Here's how the part is built. I have some questions about the finished solid (model axes, mm). Give positions to 0.01 mm unless a question says otherwise; leave off trailing zeros. Write each loop counter-clockwise with the first axis right and the second up, starting at its lowest first coordinate (ties: lowest second). Pieces come first, ordered by that corner, then holes. Notation, with made-up numbers: (-3, 67.5) -> (29, 67.5) arc R23 ccw to (29, 83.5) -> close; hole circle Ø9 at (56, -30.5). An arc over 180 degrees is marked (long way). Use one line per item in the form item = value.
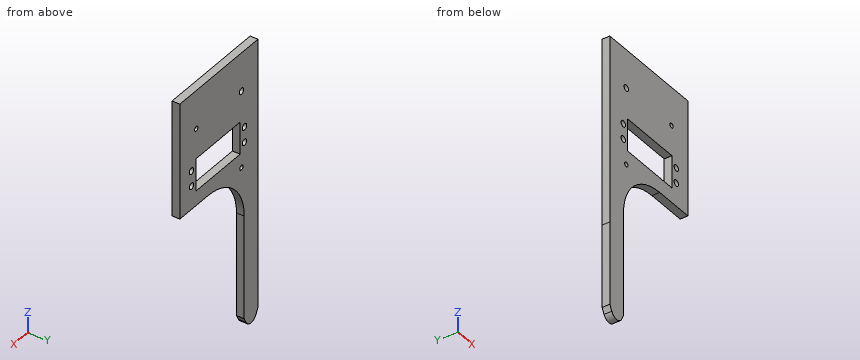
```python
from build123d import *

# Parameters (mm, degrees)
BOSS_EXTRUDE1_DEPTH = 2.5
SKETCH2_W           = 39
SKETCH2_H           = 19
CUT_EXTRUDE2_DEPTH  = 118.286651401
SKETCH6_R           = 1.5
SKETCH6_R_2         = 2
CUT_EXTRUDE11_DEPTH = 118.286651401
SKETCH8_W           = 39.164697568
SKETCH8_H           = 2
CUT_EXTRUDE12_DEPTH = 10
SKETCH9_W           = 40.5
SKETCH9_H           = 21
CUT_EXTRUDE14_DEPTH = 10
SKETCH10_R          = 2
CUT_EXTRUDE16_DEPTH = 10
SKETCH14_W          = 61.515702129
SKETCH14_H          = 51.963385976
CUT_EXTRUDE19_DEPTH = 10
FILLET4_R           = 5


with BuildPart() as part:
    # Sketch1 → Boss-Extrude1 (new, symmetric)
    with BuildSketch(Plane(origin=(0, 0, 0), x_dir=(1, 0, 0), z_dir=(0, 1, 0))):
        with BuildLine():
            Line((-45.466733516, 13.267794591), (-45.466733516, -107.999697871))
            Line((-45.466733516, -107.999697871), (25.786244138, -107.999697871))
            Line((25.786244138, -107.999697871), (25.786244138, -33))
            Line((25.786244138, -33), (0, -33))
            ThreePointArc((0, -33), (-23.334523779, -23.334523779), (-33, 0))
            Line((-33, 0), (-33, 13.267794591))
            Line((-33, 13.267794591), (-30.215321059, 13.267794591))
            ThreePointArc((-30.215321059, 13.267794591), (-18.043874009, 27.630030958), (0, 33))
            Line((0, 33), (0, 48))
            ThreePointArc((0, 48), (-17.760506671, 44.593322401), (-33, 34.856850116))
            Line((-33, 34.856850116), (-33, 66.974298245))
            Line((-33, 66.974298245), (-39.23, 79.434298245))
            Line((-39.23, 79.434298245), (-45.46, 66.974298245))
            Line((-45.46, 66.974298245), (-45.46, 13.267794591))
            Line((-45.46, 13.267794591), (-45.466733516, 13.267794591))
        make_face()
        with BuildLine():
            ThreePointArc((0, -48), (-3.55792227, -47.867955765), (-7.096269411, -47.472549547))
            Line((-7.096269411, -47.472549547), (0, -47.472549547))
            Line((0, -47.472549547), (0, -48))
        make_face(mode=Mode.SUBTRACT)
    extrude(amount=BOSS_EXTRUDE1_DEPTH, both=True)

    # Sketch2 → Cut-Extrude2 (cut, through all)
    with BuildSketch(Plane(origin=(0, 2.5, 0), x_dir=(1, 0, 0), z_dir=(0, 1, 0))):
        with Locations((-9.786245396, -52.095481266)):
            Rectangle(SKETCH2_W, SKETCH2_H)
    extrude(amount=-CUT_EXTRUDE2_DEPTH, mode=Mode.SUBTRACT)

    # Sketch6 → Cut-Extrude11 (cut, through all)
    with BuildSketch(Plane(origin=(0, 2.5, 0), x_dir=(1, 0, 0), z_dir=(0, 1, 0))):
        with Locations(Location((10.786244138, -82.999697871, 0), (0, 0, 270))):
            Circle(SKETCH6_R)
        with Locations(Location((-30.466733516, -82.999697871, 0), (0, 0, 270))):
            Circle(SKETCH6_R_2)
        with Locations(Location((-30.466733516, -33.095481266, 0), (0, 0, 270))):
            Circle(SKETCH6_R)
    extrude(amount=-CUT_EXTRUDE11_DEPTH, mode=Mode.SUBTRACT)

    # Sketch8 → Cut-Extrude12 (cut)
    with BuildSketch(Plane(origin=(0, 2.5, 0), x_dir=(1, 0, 0), z_dir=(0, 1, 0))):
        with Locations((-9.703896612, -62.595481266)):
            Rectangle(SKETCH8_W, SKETCH8_H)
    extrude(amount=-CUT_EXTRUDE12_DEPTH, mode=Mode.SUBTRACT)

    # Sketch9 → Cut-Extrude14 (cut)
    with BuildSketch(Plane(origin=(0, 2.5, 0), x_dir=(1, 0, 0), z_dir=(0, 1, 0))):
        with Locations((-9.036245396, -53.095481266)):
            Rectangle(SKETCH9_W, SKETCH9_H)
    extrude(amount=-CUT_EXTRUDE14_DEPTH, mode=Mode.SUBTRACT)

    # Sketch10 → Cut-Extrude16 (cut)
    with BuildSketch(Plane(origin=(0, 2.5, 0), x_dir=(1, 0, 0), z_dir=(0, 1, 0))):
        with Locations(Location((-33.206245396, -48.155481266, 0), (0, 0, 270))):
            Circle(SKETCH10_R)
        with Locations(Location((-33.206245396, -58.035481266, 0), (0, 0, 270))):
            Circle(SKETCH10_R)
        with Locations(Location((15.133754604, -58.035481266, 0), (0, 0, 270))):
            Circle(SKETCH10_R)
        with Locations(Location((15.133754604, -48.155481266, 0), (0, 0, 270))):
            Circle(SKETCH10_R)
    extrude(amount=-CUT_EXTRUDE16_DEPTH, mode=Mode.SUBTRACT)

    # Sketch14 → Cut-Extrude19 (cut)
    with BuildSketch(Plane(origin=(0, 2.5, 0), x_dir=(1, 0, 0), z_dir=(0, 1, 0))):
        with Locations((-2.242148935, 25.981692988)):
            Rectangle(SKETCH14_W, SKETCH14_H)
    extrude(amount=-CUT_EXTRUDE19_DEPTH, mode=Mode.SUBTRACT)

    # Fillet4
    fillet4_edges = [part.edges().sort_by_distance(p)[0] for p in [
        (-39.23, 0, -79.434298245),
    ]]
    fillet(fillet4_edges, radius=FILLET4_R)


solid = part.part
```
Q1. I want a section at D-D, the plane x = 19.5. Write out the boundary of the cut face in (y, z).
Result set:
outline = (-2.5, 33) -> (2.5, 33) -> (2.5, 108) -> (-2.5, 108) -> close
Q2. If I drill on line 1 along Z through (x, y) = (0, 1.15); line 2 along X through (y, z) = (0.5, -19); line 3 along Z through (x, y) = (-15.5, -2), over which ranges is the centre line in solid material (lowest first)? Write a range as from..to.
Result set:
line_1 = 33..42.6, 63.6..108
line_2 = -45.46..-33
line_3 = 29.13..42.6, 63.6..108
Q3. Will these pins go through, and if not, where does the flat tip stop? pin 1 Ø1.5 at (x, y) = (17.5, -1) entering from -Z; pin 2 Ø2.5 at (y, z) = (-0.5, -52.5) entering from -X; pin 3 Ø2.5 at (x, y) = (-6.5, 0) entering from -Z.
Result set:
pin_1 = 33
pin_2 = -45.46
pin_3 = 32.08
Q4. I want a section at B-B, the plane x = 3. Write out the boundary of the cut face in (y, z).
Result set:
outline = (-2.5, 33) -> (2.5, 33) -> (2.5, 42.6) -> (-2.5, 42.6) -> close; (-2.5, 63.6) -> (2.5, 63.6) -> (2.5, 108) -> (-2.5, 108) -> close
Q5. I want a section at C-C, the plane y = -1.25. Count the separate pieces of the cut face and the enclosed holes in it, and give its area (3 significant figures).
Result set:
separate_pieces = 1
enclosed_holes = 8
area = 5,950 mm2
Q6. I want a section at A-A, the plane z = 54. Write out the boundary of the cut face in (x, y).
Result set:
outline = (-45.47, -2.5) -> (-29.29, -2.5) -> (-29.29, 2.5) -> (-45.47, 2.5) -> close; (11.21, -2.5) -> (25.79, -2.5) -> (25.79, 2.5) -> (11.21, 2.5) -> close
